Verification items for the finished model (mm, model axes). A direction names the side the tool comes from. Coordinates: 2 decimals unless noted, no trailing zeros. Order: outer loops, then holes, each group sorted by start corner. A loop starts at its lowest first (then second) coordinate and runs counter-clockwise, first axis right, second up. Notation, with made-up numbers: M 45.25,88 L 69.25,88 A25 ccw 69.25,121 Z; hole C -38,23.25 d2. An arc over 180 degrees is marked long. Return JSON: item names as keys, results as strings.
```python
from build123d import *

# Parameters (mm, degrees)
SKETCH1_R           = 3.175
BOSS_EXTRUDE1_DEPTH = 12.7
SKETCH3_R           = 3.96875
BOSS_EXTRUDE2_DEPTH = 12.7
SKETCH4_R           = 1.5875
CUT_EXTRUDE2_DEPTH  = 8.89
SKETCH5_R           = 0.79375
CUT_EXTRUDE3_DEPTH  = 4.96875


with BuildPart() as part:
    # Sketch1 → Boss-Extrude1 (new body)
    with BuildSketch(Plane.XY):
        Circle(SKETCH1_R)
    extrude(amount=BOSS_EXTRUDE1_DEPTH)

    # Sketch3 → Boss-Extrude2 (add)
    with BuildSketch(Plane(origin=(0, 0, 0), x_dir=(-1, 0, 0), z_dir=(0, 0, -1))):
        Circle(SKETCH3_R)
    extrude(amount=BOSS_EXTRUDE2_DEPTH)

    # Sketch4 → Cut-Extrude2 (cut)
    with BuildSketch(Plane(origin=(0, 0, -12.7), x_dir=(-1, 0, 0), z_dir=(0, 0, -1))):
        Circle(SKETCH4_R)
    extrude(amount=-CUT_EXTRUDE2_DEPTH, mode=Mode.SUBTRACT)

    # Sketch5 → Cut-Extrude3 (cut, through all)
    with BuildSketch(Plane(origin=(0, 0, 0), x_dir=(1, 0, 0), z_dir=(0, 1, 0))):
        with Locations((0, 7.62)):
            Circle(SKETCH5_R)
    extrude(amount=CUT_EXTRUDE3_DEPTH, mode=Mode.SUBTRACT)


solid = part.part
```
Q1. Cross-section at B-B, the plane y = 0. Record the boundary of the cut face in (x, z) (1 decimal), and give its area (3 significant figures).
Values:
{"outline": "M -4,-12.7 L -1.6,-12.7 L -1.6,-3.8 L 1.6,-3.8 L 1.6,-12.7 L 4,-12.7 L 4,0 L 3.2,0 L 3.2,12.7 L -3.2,12.7 L -3.2,0 L -4,0 Z", "area": "153 mm^2"}
Q2. Cross-section at D-D, the plane y = 2.5. Record the boundary of the cut face in (x, z).
Values:
{"outline": "M -3.08,-12.7 L 3.08,-12.7 L 3.08,0 L 1.96,0 L 1.96,12.7 L -1.96,12.7 L -1.96,0 L -3.08,0 Z; hole C 0,-7.62 d1.59"}
Q3. Cross-section at C-C, the plane z = 4. Record the boundary of the cut face in (x, y) (3 decimals).
Values:
{"outline": "C 0,0 d6.35"}
Q4. Draft check along X on faces 1 (the face through (-2, 0, -12.7)), 2 (the face through (-0.793, 2.655, -7.655)), 3 (the face through (-0.69, -3.1, 6.26)). Enter one of: pulls with the +X half, pulls with the -X half, needs draft (parallel to the pull), parting line crosses it, or undercut.
Values:
{"face 1": "needs draft", "face 2": "undercut", "face 3": "parting line crosses it"}
Q5. Tool access check on faces 4 (the face through (2, 3, 0)), 5 (the face through (0.34, -1.55, -8.32)), 6 (the face through (0, 0, 12.7)). Record the directions out of +Z, -Z, +X, -X, +Y, -Y that give a thin tool (end or side, any length) a straight path to the whole face; none if there is none.
Values:
{"face 4": "+Z", "face 5": "-Z", "face 6": "+Z, +X, -X, +Y, -Y"}
Q6. Go/stop test with flat-tipped pins: pin 1 (3.5 mm diameter, centred on x = 0.5, y = 0.5, fed in from -Z); pin 2 (1.3 mm diameter, centred on x = 0, z = -7.62, fed in from +Y); pin 3 (1.9 mm diameter, centred on x = 0, y = 0, fed in from -Z); pin 4 (1 mm diameter, centred on y = 0, z = 1, fed in from +X) (3 decimals). Record where each tip stops, or that it passes through.
Values:
{"pin 1": "z = -12.7", "pin 2": "y = -1.45", "pin 3": "z = -3.81", "pin 4": "x = 3.175"}
Q7. Cross-section at A-A, the plane x = 0. Record the boundary of the cut face in (y, z) (1 decimal), and give its area (3 significant figures).
Values:
{"outline": "M -4,-12.7 L -1.6,-12.7 L -1.6,-3.8 L 1.6,-3.8 L 1.6,-6.8 L 4,-6.8 L 4,0 L 3.2,0 L 3.2,12.7 L -3.2,12.7 L -3.2,0 L -4,0 Z; M 1.6,-12.7 L 4,-12.7 L 4,-8.4 L 1.6,-8.4 Z", "area": "149 mm^2"}
Q8. Material ranges on line 1 along Y through (x, z) = (0, -9.5); line 2 along Z through (x, y) = (0, 2.85); line 3 along Z through (x, y) = (0, 3.25), recorded low to high.
Values:
{"line 1": "-3.97 to -1.59, 1.59 to 3.97", "line 2": "-12.7 to -8.41, -6.83 to 12.7", "line 3": "-12.7 to -8.41, -6.83 to 0"}
